Part print with two shaded views. Sizes in mm from the minimum x, y, z corner. Round coordinates to 2 decimals unless told otherwise and drop trailing zeros. Loops run counter-clockwise (first coordinate to the right, second up) from the corner with the lowest first, then second, coordinate; pieces in that order, holes last.
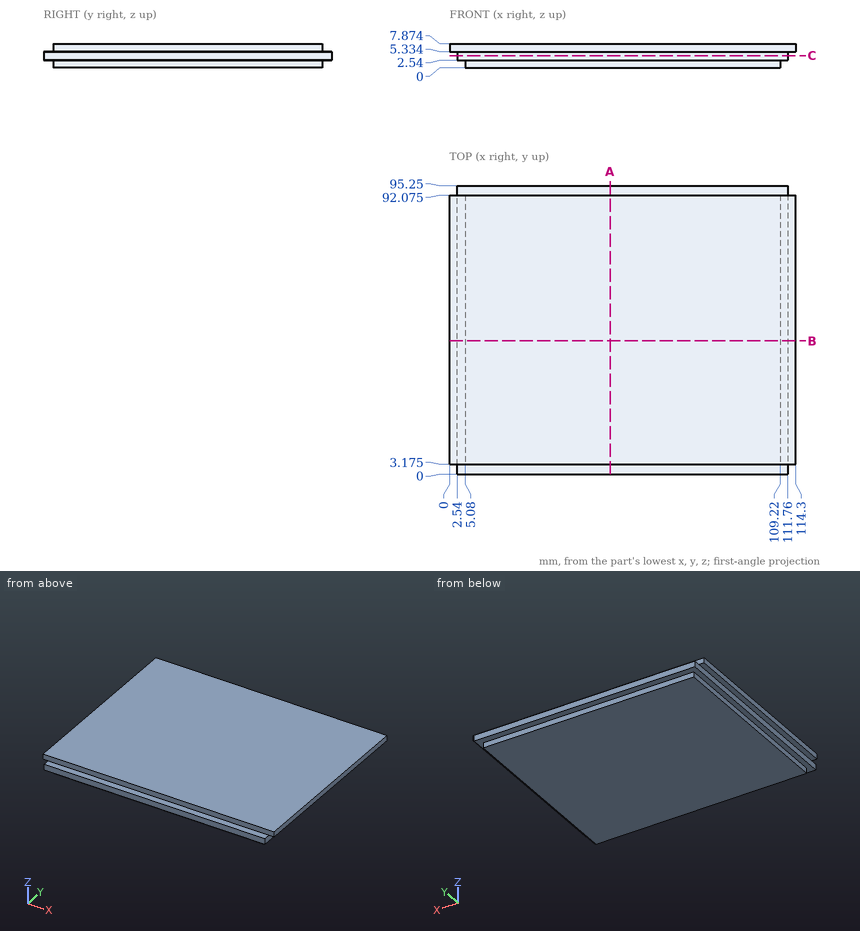
Item 1: Cut at A-A (x = 53). List the corners of the cut face in (y, z) (3 decimals), plus the area to 3 significant figures.
Verdict:
outline: (0, 2.54) - (3.175, 2.54) - (3.175, 0) - (92.075, 0) - (92.075, 2.54) - (95.25, 2.54) - (95.25, 5.334) - (92.075, 5.334) - (92.075, 7.874) - (3.175, 7.874) - (3.175, 5.334) - (0, 5.334) - close
area: 718 mm2
Item 2: Cut at C-C (z = 4). List the corners of the cut face in (x, y), plus the area to 3 significant figures.
Verdict:
outline: (2.54, 0) - (111.76, 0) - (111.76, 95.25) - (2.54, 95.25) - close
area: 10,400 mm2
Item 3: Flat gauge pins, fed straight in: P1, Ø1.3, axis at x = 113.5, y = 28.5, coming from the -Z side; P2, Ø2, axis at x = 39.5, z = 7, coming from the -Y side (3 decimals); P3, Ø1.4, axis at y = 31, z = 4, coming from the -X side; P4, Ø1, axis at x = 74.5, y = 11, coming from the -Z side. Where does each tip first touch, or does it go through?
Verdict:
P1: stops at z = 5.33
P2: stops at y = 3.175
P3: stops at x = 2.54
P4: stops at z = 0
Item 4: Cut at B-B (y = 44). List the corners of the cut face in (x, z).
Verdict:
outline: (0, 5.33) - (2.54, 5.33) - (2.54, 2.54) - (5.08, 2.54) - (5.08, 0) - (109.22, 0) - (109.22, 2.54) - (111.76, 2.54) - (111.76, 5.33) - (114.3, 5.33) - (114.3, 7.87) - (0, 7.87) - close
Item 5: Wall check: L1, parallel to Y at x = 43, z = 5.75 (3 decimals); L2, parallel to X at y = 69.5, z = 1; L3, parallel to X at y = 20, z = 5.25. Give the ranges that are in metal, low to high.
Verdict:
L1: y = 3.175 to 92.075
L2: x = 5.08 to 109.22
L3: x = 2.54 to 111.76
